from build123d import *

# Parameters (mm, degrees)
SKETCH_1_W                 = 159.5
SKETCH_1_H                 = 90.2
EXTRUDE_1_DEPTH            = 50.5
CUT_EXTRUDE_1_DEPTH        = 174.275820587
SHELL_1_T                  = -1.5
SKETCH_3_W                 = 6
SKETCH_3_H                 = 6
EXTRUDE_3_DEPTH            = 1.5
EXTRUDE_4_DEPTH            = 6
MIRROR_2_COPY_1_SKETCH_W   = 6
MIRROR_2_COPY_1_SKETCH_H   = 6
MIRROR_2_COPY_1_DEPTH      = 1.5
MIRROR_2_COPY_2_DEPTH      = 6
SKETCH_6_W                 = 50.5
SKETCH_6_H                 = 12.8
CUT_EXTRUDE_2_DEPTH        = 20
CUT_EXTRUDE_3_DEPTH        = 10
PATTERN_LINEAR_1_COUNT     = 2
PATTERN_LINEAR_1_PITCH     = 53
PATTERN_LINEAR_1_COL_COUNT = 2
PATTERN_LINEAR_1_COL_PITCH = 53
SKETCH_8_W                 = 2.45
SKETCH_8_H                 = 1.5
EXTRUDE_5_DEPTH            = 16
SKETCH_9_W                 = 156.5
SKETCH_9_H                 = 22.55
CUT_EXTRUDE_4_DEPTH        = 4.5
MIRROR_3_COPY_1_DEPTH      = 10
MIRROR_3_COPY_2_DEPTH      = 10
SKETCH_10_W                = 159.5
SKETCH_10_H                = 45.1
EXTRUDE_6_DEPTH            = 4
SKETCH_11_W                = 156.5
SKETCH_11_H                = 42.1
CUT_EXTRUDE_6_DEPTH        = 2.5
SKETCH_12_W                = 150.5
SKETCH_12_H                = 38.1
CUT_EXTRUDE_7_DEPTH        = 4
SKETCH_13_W                = 4
SKETCH_13_H                = 6.2
SKETCH_13_W_2              = 6.2
SKETCH_13_H_2              = 4
CUT_EXTRUDE_8_DEPTH        = 4


with BuildPart() as part:
    # Эскиз1 → Бобышка-Вытянуть1 (new body)
    with BuildSketch(Plane(origin=(0, 0, 0), x_dir=(1, 0, 0), z_dir=(0, 1, 0))):
        Rectangle(SKETCH_1_W, SKETCH_1_H)
    extrude(amount=EXTRUDE_1_DEPTH)

    # Эскиз2 → Вырез-Вытянуть1 (cut, through all)
    with BuildSketch(Plane(origin=(79.75, 0, 0), x_dir=(0, 0, -1), z_dir=(1, 0, 0))):
        Polygon((-46.1, 19), (-30.8, 19), (-30.8, 41), (-22.55, 41), (-22.55, 51.5), (22.55, 51.5), (22.55, 41), (30.8, 41), (30.8, 19), (46.1, 19), (46.1, 52.5), (-46.1, 52.5), align=None)
    extrude(amount=-CUT_EXTRUDE_1_DEPTH, mode=Mode.SUBTRACT)

    # Оболочка1
    shell_1_openings = [part.faces().sort_by_distance(p)[0] for p in [
        (0, 0, 0),
    ]]
    offset(amount=SHELL_1_T, openings=shell_1_openings, kind=Kind.INTERSECTION)

    # Эскиз3 → Бобышка-Вытянуть3 (add)
    with BuildSketch(Plane(origin=(79.75, 0, 0), x_dir=(0, 0, -1), z_dir=(1, 0, 0))):
        with Locations((-35.6, -3)):
            Rectangle(SKETCH_3_W, SKETCH_3_H)
    extrude_3 = extrude(amount=-EXTRUDE_3_DEPTH)

    # Эскиз4 → Бобышка-Вытянуть4 (add)
    with BuildSketch(Plane.XY.offset(38.6)):
        Polygon((78.25, -6), (77.25, -4.4), (77.25, -4), (78.75, -4), (78.75, -6), align=None)
    extrude_4 = extrude(amount=-EXTRUDE_4_DEPTH)

    # Зеркальное отражение1: Бобышка-Вытянуть3, Бобышка-Вытянуть4 across plane
    add(extrude_3.mirror(Plane.XY))
    add(extrude_4.mirror(Plane.XY))

    # Зеркальное отражение2: Бобышка-Вытянуть3, Бобышка-Вытянуть4 across plane
    add(extrude_3.mirror(Plane(origin=(0, 0, 0), x_dir=(0, 0, 1), z_dir=(1, 0, 0))))
    add(extrude_4.mirror(Plane(origin=(0, 0, 0), x_dir=(0, 0, 1), z_dir=(1, 0, 0))))

    # Зеркальное отражение2 copy 1 sketch → Зеркальное отражение2 copy 1 (add)
    with BuildSketch(Plane.ZY.offset(79.75)):
        with Locations((-35.6, -3)):
            Rectangle(MIRROR_2_COPY_1_SKETCH_W, MIRROR_2_COPY_1_SKETCH_H)
    extrude(amount=-MIRROR_2_COPY_1_DEPTH)

    # Зеркальное отражение2 copy 2 sketch → Зеркальное отражение2 copy 2 (add)
    with BuildSketch(Plane(origin=(0, 0, -38.6), x_dir=(-1, 0, 0), z_dir=(0, 0, -1))):
        Polygon((78.25, -6), (77.25, -4.4), (77.25, -4), (78.75, -4), (78.75, -6), align=None)
    extrude(amount=-MIRROR_2_COPY_2_DEPTH)

    # Эскиз6 → Вырез-Вытянуть2 (cut)
    with BuildSketch(Plane(origin=(0, 19, 0), x_dir=(1, 0, 0), z_dir=(0, 1, 0))):
        with Locations((0, -37.2)):
            Rectangle(SKETCH_6_W, SKETCH_6_H)
        with Locations((-53, -37.2)):
            Rectangle(SKETCH_6_W, SKETCH_6_H)
        with Locations((53, -37.2)):
            Rectangle(SKETCH_6_W, SKETCH_6_H)
    cut_extrude_2 = extrude(amount=-CUT_EXTRUDE_2_DEPTH, mode=Mode.SUBTRACT)

    # Эскиз7 → Вырез-Вытянуть3 (cut)
    with BuildSketch(Plane.XY.offset(45.1)):
        Polygon((-22.8, 19.5), (-22.5, 6), (22.5, 6), (22.8, 19.5), align=None)
    cut_extrude_3 = extrude(amount=-CUT_EXTRUDE_3_DEPTH, mode=Mode.SUBTRACT)

    # Линейный массив1: Вырез-Вытянуть3 ×2
    with Locations(*[(i * PATTERN_LINEAR_1_PITCH, 0, 0) for i in range(1, PATTERN_LINEAR_1_COUNT)]):
        add(cut_extrude_3, mode=Mode.SUBTRACT)

    # Линейный массив1 col: Вырез-Вытянуть3 ×2
    with Locations(*[(-i * PATTERN_LINEAR_1_COL_PITCH, 0, 0) for i in range(1, PATTERN_LINEAR_1_COL_COUNT)]):
        add(cut_extrude_3, mode=Mode.SUBTRACT)

    # Эскиз8 → Бобышка-Вытянуть5 (add)
    with BuildSketch(Plane.XZ.offset(-17.5)):
        Polygon((-30.2, 30.8), (-30.2, 29.3), (-22.8, 29.3), (-22.8, 30.8), (-25.25, 30.8), (-25.25, 43.6), (-27.75, 43.6), (-27.75, 30.8), align=None)
        Polygon((22.8, 30.8), (22.8, 29.3), (30.2, 29.3), (30.2, 30.8), (27.75, 30.8), (27.75, 43.6), (25.25, 43.6), (25.25, 30.8), align=None)
        with Locations((-77.025, 30.05)):
            Rectangle(SKETCH_8_W, SKETCH_8_H)
        with Locations((77.025, 30.05)):
            Rectangle(SKETCH_8_W, SKETCH_8_H)
    extrude_5 = extrude(amount=EXTRUDE_5_DEPTH)

    # Эскиз9 → Вырез-Вытянуть4 (cut)
    with BuildSketch(Plane.XZ):
        with Locations((0, 32.325)):
            Rectangle(SKETCH_9_W, SKETCH_9_H)
    cut_extrude_4 = extrude(amount=-CUT_EXTRUDE_4_DEPTH, mode=Mode.SUBTRACT)

    # Зеркальное отражение3: Вырез-Вытянуть2, Вырез-Вытянуть3, Бобышка-Вытянуть5, Вырез-Вытянуть4 across plane
    add(cut_extrude_2.mirror(Plane.XY), mode=Mode.SUBTRACT)
    add(cut_extrude_3.mirror(Plane.XY), mode=Mode.SUBTRACT)
    add(extrude_5.mirror(Plane.XY))
    add(cut_extrude_4.mirror(Plane.XY), mode=Mode.SUBTRACT)

    # Зеркальное отражение3 copy 1 sketch → Зеркальное отражение3 copy 1 (cut)
    with BuildSketch(Plane(origin=(53, 0, -45.1), x_dir=(1, 0, 0), z_dir=(0, 0, -1))):
        Polygon((-22.8, -19.5), (-22.5, -6), (22.5, -6), (22.8, -19.5), align=None)
    extrude(amount=-MIRROR_3_COPY_1_DEPTH, mode=Mode.SUBTRACT)

    # Зеркальное отражение3 copy 2 sketch → Зеркальное отражение3 copy 2 (cut)
    with BuildSketch(Plane(origin=(-53, 0, -45.1), x_dir=(1, 0, 0), z_dir=(0, 0, -1))):
        Polygon((-22.8, -19.5), (-22.5, -6), (22.5, -6), (22.8, -19.5), align=None)
    extrude(amount=-MIRROR_3_COPY_2_DEPTH, mode=Mode.SUBTRACT)

    # Эскиз10 → Бобышка-Вытянуть6 (add)
    with BuildSketch(Plane(origin=(0, 50.5, 0), x_dir=(1, 0, 0), z_dir=(0, 1, 0))):
        Rectangle(SKETCH_10_W, SKETCH_10_H)
    extrude(amount=-EXTRUDE_6_DEPTH)

    # Эскиз11 → Вырез-Вытянуть6 (cut)
    with BuildSketch(Plane(origin=(0, 50.5, 0), x_dir=(1, 0, 0), z_dir=(0, 1, 0))):
        Rectangle(SKETCH_11_W, SKETCH_11_H)
    extrude(amount=-CUT_EXTRUDE_6_DEPTH, mode=Mode.SUBTRACT)

    # Эскиз12 → Вырез-Вытянуть7 (cut)
    with BuildSketch(Plane(origin=(0, 48, 0), x_dir=(1, 0, 0), z_dir=(0, 1, 0))):
        Rectangle(SKETCH_12_W, SKETCH_12_H)
    extrude(amount=-CUT_EXTRUDE_7_DEPTH, mode=Mode.SUBTRACT)

    # Эскиз13 → Вырез-Вытянуть8 (cut)
    with BuildSketch(Plane(origin=(0, 48, 0), x_dir=(1, 0, 0), z_dir=(0, 1, 0))):
        with Locations((-75.75, 0)):
            Rectangle(SKETCH_13_W, SKETCH_13_H)
        with Locations((0, 18.55)):
            Rectangle(SKETCH_13_W_2, SKETCH_13_H_2)
        with Locations((0, -18.55)):
            Rectangle(SKETCH_13_W_2, SKETCH_13_H_2)
        with Locations((75.75, 0)):
            Rectangle(SKETCH_13_W, SKETCH_13_H)
    extrude(amount=-CUT_EXTRUDE_8_DEPTH, mode=Mode.SUBTRACT)


solid = part.part
Work out the finished part from the listing and answer in its coordinate system (mm). A direction names the side the tool comes from. Coordinates: 2 decimals unless noted, no trailing zeros. Write each loop counter-clockwise with the first axis right and the second up, starting at its lowest first coordinate (ties: lowest second). Pieces come first, ordered by that corner, then holes. Notation, with made-up numbers: M 4,21.25 L 8,21.25 A21 ccw 8,56.25 Z; hole C 72.5,-32.5 d7. An arc over 180 degrees is marked long. Answer as CSV lines item,"result". Start each with the question number.
Item 1: Section A-A on x = 6.5 is taken. Give the number of separate pieces and of enclosed holes in the cut face, and give its area (3 significant figures).
Item 2: Flat-ended cylindrical pins translate along their axes: P1, Ø1.2, axis at x = 53.5, y = 47.5, coming from the -Z side; P2, Ø4, axis at x = 62.5, z = 30, coming from the -Y side; P3, Ø1.6, axis at x = 26, y = 47.5, coming from the +Z side. Find the tip coordinate at first contact, or state that the pin passes through.
Item 3: A tool of negligible diameter and unlimited length cuts with its end or side. For faces 1 (the face through (79.75, 22, 1)), 2 (the face through (-27, 4.5, 35)), 3 (the face through (25.25, 12, 37)), 4 (the face through (1, 41, 27)), 5 (the face through (1, 41, -27)), from which of +Z, -Z, +X, -X, +Y, -Y can it reach the whole face along a straight path? Write none if from no direction.
Item 4: Determine the mould class of faces 6 (the face through (-1, 26, -29.3)), 7 (the face through (-79.75, 22, 1)) for opening direction Z: released by +Z, released by -Z, zero draft, split by the parting line, or undercut.
Item 5: Section D-D on z = 16.5 is taken. Write down the section's boundary in (x, y), and give its area (4 significant figures).
Item 6: Section B-B on z = 37 is taken. Write down the section's boundary in (x, y), and give its area (3 significant figures).
Item 7: Consider L1, parallel to X at y = 15.5, z = -36.5; L2, parallel to Z at x = 38, y = 31; L3, parallel to X at y = 28, z = -14. Determine where each line is inside the solid, lowest interval first.
Item 8: Section C-C on y = 44 is taken. Write down the section's boundary in (x, z), and give its area (3 significant figures).
Checks:
1,separate pieces,"4"
1,enclosed holes,"0"
1,area,"148 mm²"
2,P1,"stops at z = -22.55"
2,P2,"stops at y = 17.5"
2,P3,"stops at z = 22.55"
3,face 1,"+Z, -Z, +X, +Y, -Y"
3,face 2,"-Y"
3,face 3,"+Y, -Y"
3,face 4,"+Z, +X, -X, +Y"
3,face 5,"-Z, +X, -X, +Y"
4,face 6,"undercut"
4,face 7,"zero draft"
5,outline,"M -79.75,0 L -78.25,0 L -78.25,46.5 L -75.25,46.5 L -75.25,48 L -78.25,48 L -78.25,50.5 L -79.75,50.5 Z; M 75.25,46.5 L 78.25,46.5 L 78.25,0 L 79.75,0 L 79.75,50.5 L 78.25,50.5 L 78.25,48 L 75.25,48 Z"
5,area,"160.5 mm²"
6,outline,"M -79.75,-6 L -78.25,-6 L -77.25,-4.4 L -77.25,-4 L -78.25,-4 L -78.25,19 L -79.75,19 Z; M -27.75,4.5 L -25.25,4.5 L -25.25,19 L -27.75,19 Z; M 25.25,4.5 L 27.75,4.5 L 27.75,19 L 25.25,19 Z; M 77.25,-4.4 L 78.25,-6 L 79.75,-6 L 79.75,19 L 78.25,19 L 78.25,-4 L 77.25,-4 Z"
6,area,"150 mm²"
7,L1,"x = -79.75 to -78.25, -27.75 to -25.25, 25.25 to 27.75, 78.25 to 79.75"
7,L2,"z = -30.8 to -29.3, 29.3 to 30.8"
7,L3,"x = -79.75 to -78.25, 78.25 to 79.75"
8,outline,"M -79.75,-22.55 L 79.75,-22.55 L 79.75,22.55 L -79.75,22.55 Z; hole M -78.25,-21.05 L 78.25,-21.05 L 78.25,21.05 L -78.25,21.05 Z"
8,area,"605 mm²"
